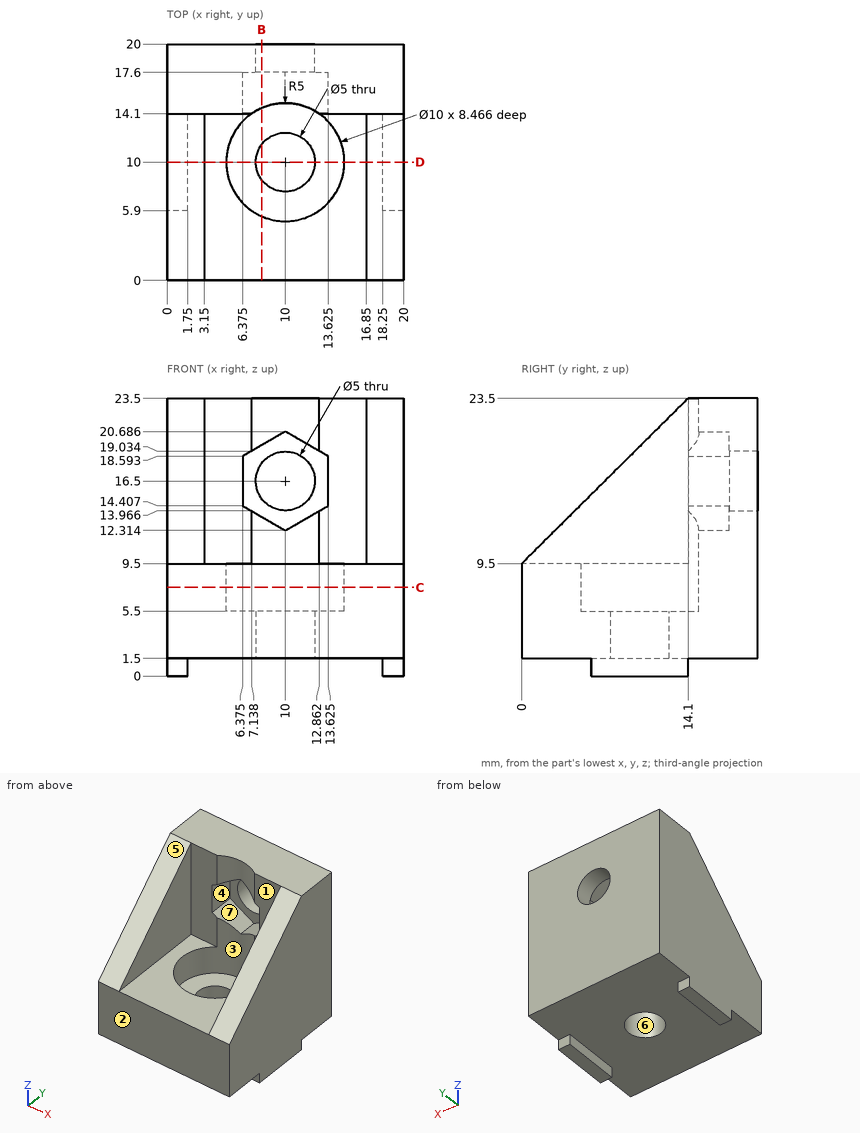
Job drawing, mm, ordinate dimensions from the low corner. One solid piece. A direction names the side the tool comes from. Round coordinates to 2 decimals unless told otherwise and drop trailing zeros. Loops run counter-clockwise (first coordinate to the right, second up) from the corner with the lowest first, then second, coordinate; pieces in that order, holes last.
Item 1: Cut at B-B, the plane x = 8. Give the cut face in (y, z), then the cut area to 3 significant figures.
Item 2: Cut at D-D, the plane y = 10. Give the cut face in (x, z), then the cut area to 3 significant figures.
Item 3: Mould opens along Z. For the marked faces 5, 6 and 7 say: +Z half, -Z half, draft (parallel to the pull), parting line (faces both ways), or undercut.
Item 4: Cut at C-C, the plane z = 7.5. Give the cut face in (x, y).
Item 5: Drop flat-ended pins along their axis: P1, Ø1.5, axis at x = 14.5, y = 13, coming from the -Z side; P2, Ø8, axis at x = 10, y = 10, coming from the +Z side; P3, Ø3.5, axis at x = 10, z = 17.5, coming from the -Y side. Give the stop position or say it passes through.
Item 6: Drill centre lines: line 1 (X direction, y = 10, z = 2.7); line 2 (X direction, y = 10, z = 7.5). Where is each one in solid material? Low to high.
Item 7: 3-axis set-ups, long thin cutter, end or side, ignore diameter. For the marked faces 1, 2, 3 and 4: which of +Z, -Z, +X, -X, +Y, -Y reach the whole face in a straight line?
A:
1. outline: (0, 1.5) - (8.5, 1.5) - (8.5, 5.5) - (5.42, 5.5) - (5.42, 9.5) - (0, 9.5) - close; (11.5, 1.5) - (20, 1.5) - (20, 15) - (17.6, 15) - (17.6, 13.47) - (14.58, 13.47) - (14.58, 5.5) - (11.5, 5.5) - close; (14.58, 19.53) - (17.6, 19.53) - (17.6, 18) - (20, 18) - (20, 23.5) - (14.58, 23.5) - close
1. area: 162 mm2
2. outline: (0, 0) - (1.75, 0) - (1.75, 1.5) - (7.5, 1.5) - (7.5, 5.5) - (5, 5.5) - (5, 9.5) - (3.15, 9.5) - (3.15, 19.43) - (0, 19.43) - close; (12.5, 1.5) - (18.25, 1.5) - (18.25, 0) - (20, 0) - (20, 19.43) - (16.85, 19.43) - (16.85, 9.5) - (15, 9.5) - (15, 5.5) - (12.5, 5.5) - close
2. area: 168 mm2
3. face 5: +Z half
3. face 6: draft
3. face 7: undercut
4. outline: (0, 0) - (20, 0) - (20, 20) - (0, 20) - close; hole circle Ø10 at (10, 10)
5. P1: stops at z = 1.5
5. P2: stops at z = 5.5
5. P3: stops at y = 17.6
6. line 1: x = 0 to 7.5, 12.5 to 20
6. line 2: x = 0 to 5, 15 to 20
7. face 1: +Z, -Y
7. face 2: +Z, -Z, +X, -X, -Y
7. face 3: +Z
7. face 4: -Y
